Could you check a few things on this model? Use its own coordinates, in mm. Face numbers are marked on the shaded views. A direction names the side the tool comes from. Coordinates: 2 decimals unless noted, no trailing zeros. Order: outer loops, then holes, each group sorted by start corner. A loop starts at its lowest first (then second) coordinate and runs counter-clockwise, first axis right, second up. Notation, with made-up numbers: (0.25, 88.5) - (23.25, 88.5) arc R18 ccw to (23.25, 115.5) - close; hole circle Ø6 at (-24, -16.75). An arc over 180 degrees is marked (long way). One line per item, written item: value. Start each with the question number.
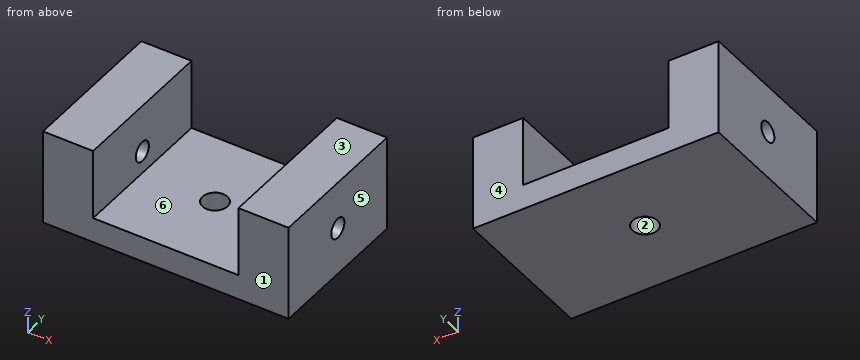
from build123d import *

# Parameters (mm, degrees)
F0_W     = 29
F0_H     = 30
F0_R     = 2.5
F1_DEPTH = 5
F0_W_2   = 10
F2_DEPTH = 19
F3_DEPTH = 19
F4_R     = 2
F5_DEPTH = 49.001


with BuildPart() as f1:
    # F0 (on Top) → F1 (new body)
    with BuildSketch(Plane.XY):
        Rectangle(F0_W, F0_H)
        Circle(F0_R, mode=Mode.SUBTRACT)
    extrude(amount=F1_DEPTH)

    # F0 (on Top) → F2 (join)
    with BuildSketch(Plane.XY):
        with Locations((-19.5, 0)):
            Rectangle(F0_W_2, F0_H)
    extrude(amount=F2_DEPTH)

    # F0 (on Top) → F3 (join)
    with BuildSketch(Plane.XY):
        with Locations((19.5, 0)):
            Rectangle(F0_W_2, F0_H)
    extrude(amount=F3_DEPTH)

    # F4 (on face) → F5 (cut, through all)
    with BuildSketch(Plane.YZ.offset(24.5)):
        with Locations((0, 9.5)):
            Circle(F4_R)
    extrude(amount=-F5_DEPTH, mode=Mode.SUBTRACT)


solid = f1.part
Q1. I'm going to push flat-ended pins straight in: pin 1 (8 mm diameter, centred on x = 9, y = 10, fed in from +Z); pin 2 (6.5 mm diameter, centred on y = 0, z = 9.5, fed in from +X). Where does each tip first touch, or does it pass through?
Q2. I want a section at C-C on z = 6.25. Please give me the cut outline in (x, y), then the cut area to 3 significant figures.
Q3. We'd pull the mould along Y, two halves only. Please class the marked faces 1, 2, 3 and 4: +Y half, -Y half, draft (parallel to the pull), parting line (faces both ways), or undercut.
Q4. If I drill on L1, parallel to X at y = -11.5, z = 15.5; L2, parallel to Y at x = 0, z = 2.9; L3, parallel to Z at x = 17.75, y = 0, over which ranges is the centre line in solid material (lowest first)?
Q5. I want a section at D-D on x = 20. Please give me the cut outline in (y, z), then the cut area to 3 significant figures.
Q6. I want a section at B-B on y = 0. Please give me the cut outline in (x, z), then the cut area to 3 significant figures.
Q7. Which directions (+Z, -Z, +X, -X, +Y, -Y) give clear straight access to the entire face, cutting with the end or side of a thin tool? Please do the marked faces 5 and 6.
Q8. I want a section at A-A on x = 0. Please give me the cut outline in (y, z).
Values follow:
1. pin 1: stops at z = 5
1. pin 2: stops at x = 24.5
2. outline: (-24.5, -15) - (-14.5, -15) - (-14.5, 15) - (-24.5, 15) - close; (14.5, -15) - (24.5, -15) - (24.5, 15) - (14.5, 15) - close
2. area: 600 mm^2
3. face 1: -Y half
3. face 2: undercut
3. face 3: draft
3. face 4: +Y half
4. L1: x = -24.5 to -14.5, 14.5 to 24.5
4. L2: y = -15 to -2.5, 2.5 to 15
4. L3: z = 0 to 7.5, 11.5 to 19
5. outline: (-15, 0) - (15, 0) - (15, 19) - (-15, 19) - close; hole circle Ø4 at (0, 9.5)
5. area: 557 mm^2
6. outline: (-24.5, 0) - (-2.5, 0) - (-2.5, 5) - (-14.5, 5) - (-14.5, 7.5) - (-24.5, 7.5) - close; (-24.5, 11.5) - (-14.5, 11.5) - (-14.5, 19) - (-24.5, 19) - close; (2.5, 0) - (24.5, 0) - (24.5, 7.5) - (14.5, 7.5) - (14.5, 5) - (2.5, 5) - close; (14.5, 11.5) - (24.5, 11.5) - (24.5, 19) - (14.5, 19) - close
6. area: 420 mm^2
7. face 5: +Z, -Z, +X, +Y, -Y
7. face 6: +Z, +Y, -Y
8. outline: (-15, 0) - (-2.5, 0) - (-2.5, 5) - (-15, 5) - close; (2.5, 0) - (15, 0) - (15, 5) - (2.5, 5) - close
